```python
from build123d import *

# Parameters (mm, degrees)
SKETCH_1_W          = 16
SKETCH_1_H          = 2
EXTRUDE_1_DEPTH     = 30
FILLET_1_R          = 8
FILLET_2_R          = 8
SKETCH_2_W          = 16
SKETCH_2_H          = 2
EXTRUDE_2_DEPTH     = 32
FILLET_3_R          = 8
FILLET_4_R          = 8
SKETCH_4_R          = 2.5
CUT_EXTRUDE_2_DEPTH = 2
SKETCH_3_R          = 2.5
CUT_EXTRUDE_3_DEPTH = 2


with BuildPart() as part:
    # 草图1 → 凸台-拉伸1 (new body)
    with BuildSketch(Plane.XY):
        with Locations((8, 1)):
            Rectangle(SKETCH_1_W, SKETCH_1_H)
    extrude(amount=EXTRUDE_1_DEPTH)

    # 圆角1
    fillet_1_edges = [part.edges().sort_by_distance(p)[0] for p in [
        (0, 1, 30),
    ]]
    fillet(fillet_1_edges, radius=FILLET_1_R)

    # 圆角2
    fillet_2_edges = [part.edges().sort_by_distance(p)[0] for p in [
        (16, 1, 30),
    ]]
    fillet(fillet_2_edges, radius=FILLET_2_R - 0.0001)  # a hair under: the kernel refuses the full size

    # 草图2 → 凸台-拉伸2 (add)
    with BuildSketch(Plane(origin=(0, 0, 0), x_dir=(1, 0, 0), z_dir=(0, 1, 0))):
        with Locations((8, 1)):
            Rectangle(SKETCH_2_W, SKETCH_2_H)
    extrude(amount=EXTRUDE_2_DEPTH)

    # 圆角3
    fillet_3_edges = [part.edges().sort_by_distance(p)[0] for p in [
        (16, 32, -1),
    ]]
    fillet(fillet_3_edges, radius=FILLET_3_R)

    # 圆角4
    fillet_4_edges = [part.edges().sort_by_distance(p)[0] for p in [
        (0, 32, -1),
    ]]
    fillet(fillet_4_edges, radius=FILLET_4_R - 0.0001)  # a hair under: the kernel refuses the full size

    # 草图4 → 切除-拉伸2 (cut)
    with BuildSketch(Plane(origin=(0, 2, 0), x_dir=(1, 0, 0), z_dir=(0, 1, 0))):
        with Locations(Location((8, -22, 0), (0, 0, 270))):
            Circle(SKETCH_4_R)
    extrude(amount=-CUT_EXTRUDE_2_DEPTH, mode=Mode.SUBTRACT)

    # 草图3 → 切除-拉伸3 (cut)
    with BuildSketch(Plane.XY):
        with Locations((8, 24)):
            Circle(SKETCH_3_R)
        with Locations((8, 40)):
            Circle(SKETCH_3_R)
    extrude(amount=-CUT_EXTRUDE_3_DEPTH, mode=Mode.SUBTRACT)


solid = part.part
```
Geometry: final body of the model. Coordinates: model frame, mm. A direction names the side the tool comes from. Give positions to 0.01 mm unless a question says otherwise; leave off trailing zeros. Loops run counter-clockwise (first coordinate to the right, second up) from the corner with the lowest first, then second, coordinate; pieces in that order, holes last. Notation, with made-up numbers: (58, 73.25) -> (116, 73.25) arc R6 cw to (116, 81.25) -> close; hole circle Ø9 at (39.5, 9.5). An arc over 180 degrees is marked (long way). Return JSON: item names as keys, results as strings.
Item 1: Pin query (flat end, axial travel): P1, Ø5, axis at x = 11, z = 15, coming from the +Y side; P2, Ø6, axis at x = 8, y = 24, coming from the +Z side. Return the tip coordinate at first contact, or that it passes through.
Filled in:
{"P1": "y = 2", "P2": "z = 0"}
Item 2: Access query for faces 4 (the flat face through (8, 2, 15)), 5 (the cylindrical face through (2.406, 29.719, -1.014)). Directions: +Z, -Z, +X, -X, +Y, -Y. A direction counts if a zero-diameter tool reaches every point of the face in a straight line with its end or side. Return the directions, or none.
Filled in:
{"face 4": "+Z, +X, -X, +Y", "face 5": "+Z, -Z, -X, +Y"}
Item 3: Section A-A, the plane z = 20.5. Output: boundary loops of the cut face in (x, y).
Filled in:
{"outline": "(0, 0) -> (6, 0) -> (6, 2) -> (0, 2) -> close; (10, 0) -> (16, 0) -> (16, 2) -> (10, 2) -> close"}
Item 4: Mould query, pull axis X, two halves, no side actions, for faces 1 (the cylindrical face through (6.5, 1, 20)), 2 (the cylindrical face through (2.281, 1.014, 27.594)), 3 (the flat face through (16, 1, 5)). Classes: released by +X, released by -X, zero draft, split by the parting line, or undercut.
Filled in:
{"face 1": "undercut", "face 2": "released by -X", "face 3": "released by +X"}
Item 5: Section C-C, the plane y = 3.5. Output: boundary loops of the cut face in (x, z), plus the area to 3 significant figures.
Filled in:
{"outline": "(0, -2) -> (16, -2) -> (16, 0) -> (0, 0) -> close", "area": "32.0 mm^2"}
Item 6: Section D-D, the plane x = 12.5. Output: boundary loops of the cut face in (y, z).
Filled in:
{"outline": "(0, -2) -> (30.61, -2) -> (30.61, 0) -> (2, 0) -> (2, 28.61) -> (0, 28.61) -> close"}
Item 7: Line query: line 1 (X direction, y = 1, z = 22); line 2 (Z direction, x = 14, y = 16); line 3 (Y direction, x = 3, z = 24.5). Output: solid intervals per line, ascending.
Filled in:
{"line 1": "0 to 5.5, 10.5 to 16", "line 2": "-2 to 0", "line 3": "0 to 2"}
Item 8: Section B-B, the plane x = 7. Output: boundary loops of the cut face in (y, z), plus the area to 3 significant figures.
Filled in:
{"outline": "(0, -2) -> (21.71, -2) -> (21.71, 0) -> (2, 0) -> (2, 19.71) -> (0, 19.71) -> close; (0, 24.29) -> (2, 24.29) -> (2, 29.94) -> (0, 29.94) -> close; (26.29, -2) -> (31.94, -2) -> (31.94, 0) -> (26.29, 0) -> close", "area": "105 mm^2"}
